```python
from build123d import *

# Parameters (mm, degrees)
ESQUISSE1_R             = 2.19
BOSS_EXTRU_2_DEPTH      = 3
ESQUISSE1_W             = 22.82
ESQUISSE1_H             = 8.5
BOSS_EXTRU_2_2_DEPTH    = 3
BOSS_EXTRU_4_DEPTH      = 3
CONG_1_R                = 3
ESQUISSE4_W             = 3
ESQUISSE4_H             = 9.614426754
BOSS_EXTRU_5_DEPTH      = 5
ENL_V_MAT_EXTRU_1_DEPTH = 5
ESQUISSE15_W            = 3
ESQUISSE15_H            = 34.885573246
BOSS_EXTRU_6_DEPTH      = 22.8
ESQUISSE17_R            = 1.25
ENL_V_MAT_EXTRU_2_DEPTH = 4
ESQUISSE19_R            = 2.5
ENL_V_MAT_EXTRU_5_DEPTH = 4


with BuildPart() as part:
    # Esquisse1 → Boss.-Extru.2 (new body)
    with BuildSketch(Plane.XY):
        Polygon((-22.134709342, 12.031312967), (-22.134709342, 3.531312967), (-2.314709342, 3.531312967), (-2.314709342, 2.416886213), (0.685290658, 2.416886213), (0.685290658, 12.031312967), align=None)
        with Locations((-17.224709342, 6.731312967)):
            Circle(ESQUISSE1_R, mode=Mode.SUBTRACT)
        with Locations((-7.224709342, 6.731312967)):
            Circle(ESQUISSE1_R, mode=Mode.SUBTRACT)
    extrude(amount=BOSS_EXTRU_2_DEPTH)



with BuildPart() as body_2:
    # Esquisse1 → Boss.-Extru.2 2 (new body)
    with BuildSketch(Plane.XY):
        with Locations((-10.724709342, -42.718687033)):
            Rectangle(ESQUISSE1_W, ESQUISSE1_H)
        with Locations((-17.224709342, -41.668687033)):
            Circle(ESQUISSE1_R, mode=Mode.SUBTRACT)
        with Locations((-7.224709342, -41.668687033)):
            Circle(ESQUISSE1_R, mode=Mode.SUBTRACT)
    extrude(amount=BOSS_EXTRU_2_2_DEPTH)

    # Esquisse3 → Boss.-Extru.4 (add)
    with BuildSketch(Plane(origin=(0.685290658, 0, 0), x_dir=(0, 0, -1), z_dir=(1, 0, 0))):
        with BuildLine():
            Line((0, 2.416886213), (0, 12.031312967))
            Line((0, 12.031312967), (-31.7, 12.031312967))
            Line((-31.7, 12.031312967), (-31.7, -46.968687033))
            Line((-31.7, -46.968687033), (0, -46.968687033))
            Line((0, -46.968687033), (0, -38.468687033))
            Line((0, -38.468687033), (-3, -38.468687033))
            ThreePointArc((-3, -38.468687033), (-4.5, -36.968687033), (-3, -35.468687033))
            Line((-3, -35.468687033), (5, -35.468687033))
            Line((5, -35.468687033), (5, -0.583113787))
            Line((5, -0.583113787), (-3, -0.583113787))
            ThreePointArc((-3, -0.583113787), (-4.5, 0.916886213), (-3, 2.416886213))
            Line((-3, 2.416886213), (0, 2.416886213))
        make_face()
    extrude(amount=BOSS_EXTRU_4_DEPTH)

    # Congé1
    cong_1_edges = [body_2.edges().sort_by_distance(p)[0] for p in [
        (2.185290658, -35.468687033, -5),
        (2.185290658, -0.583113787, -5),
    ]]
    fillet(cong_1_edges, radius=CONG_1_R)


with BuildPart() as part_1:
    add(part.part)

    add(body_2.part)  # Boss.-Extru.5 merges body 2
    # Esquisse4 → Boss.-Extru.5 (add)
    with BuildSketch(Plane(origin=(3.685290658, 0, 0), x_dir=(0, 0, -1), z_dir=(1, 0, 0))):
        with Locations((-1.5, 7.22409959)):
            Rectangle(ESQUISSE4_W, ESQUISSE4_H)
    extrude(amount=-BOSS_EXTRU_5_DEPTH)

    # Esquisse13 → Enlèv. mat.-Extru.1 (cut)
    with BuildSketch(Plane.ZY.offset(-0.685290658)):
        Polygon((28.7, -0.583113787), (31.7, -0.583113787), (31.7, 12.031312967), (24.585573245, 12.031312967), (24.585573245, 3.531312967), (28.7, 3.531312967), align=None)
        with BuildLine():
            ThreePointArc((28.7, -0.583113787), (25.790660941, 0.621973908), (24.585573245, 3.531312967))
            Line((24.585573245, 3.531312967), (28.7, 3.531312967))
            Line((28.7, 3.531312967), (28.7, -0.583113787))
        make_face()
        Polygon((31.7, -46.968687033), (31.7, -35.468687033), (28.7, -35.468687033), (28.7, -38.468687033), (25.7, -38.468687033), (25.7, -46.968687033), align=None)
        with BuildLine():
            ThreePointArc((25.7, -38.468687033), (26.578679656, -36.347366689), (28.7, -35.468687033))
            Line((28.7, -35.468687033), (28.7, -38.468687033))
            Line((28.7, -38.468687033), (25.7, -38.468687033))
        make_face()
    extrude(amount=-ENL_V_MAT_EXTRU_1_DEPTH, mode=Mode.SUBTRACT)

    # Esquisse15 → Boss.-Extru.6 (add)
    with BuildSketch(Plane.ZY.offset(-0.685290658)):
        with Locations((30.2, -18.02590041)):
            Rectangle(ESQUISSE15_W, ESQUISSE15_H)
    extrude(amount=BOSS_EXTRU_6_DEPTH)

    # Esquisse17 → Enlèv. mat.-Extru.2 (cut)
    with BuildSketch(Plane(origin=(3.685290658, 0, 0), x_dir=(0, 0, -1), z_dir=(1, 0, 0))):
        with Locations((-20.861566887, -16.89090041)):
            Circle(ESQUISSE17_R)
        with Locations((-20.861566887, -24.89090041)):
            Circle(ESQUISSE17_R)
        with Locations((-12.861566887, -24.89090041)):
            Circle(ESQUISSE17_R)
        with Locations((-4.861566887, -24.89090041)):
            Circle(ESQUISSE17_R)
        with Locations((-4.861566887, -16.89090041)):
            Circle(ESQUISSE17_R)
        with Locations((-4.861566887, -8.89090041)):
            Circle(ESQUISSE17_R)
        with Locations((-12.861566887, -8.89090041)):
            Circle(ESQUISSE17_R)
        with Locations((-20.861566887, -8.89090041)):
            Circle(ESQUISSE17_R)
        with Locations((-12.861566887, -0.89090041)):
            Circle(ESQUISSE17_R)
        with Locations((-12.861566887, -32.89090041)):
            Circle(ESQUISSE17_R)
        with Locations((-12.861566887, -16.89090041)):
            Circle(ESQUISSE17_R)
    extrude(amount=-ENL_V_MAT_EXTRU_2_DEPTH, mode=Mode.SUBTRACT)

    # Esquisse19 → Enlèv. mat.-Extru.5 (cut)
    with BuildSketch(Plane.XY.offset(31.7)):
        with Locations((-12.214709342, -6.873113787)):
            Circle(ESQUISSE19_R)
        with Locations((-12.214709342, -29.178687033)):
            Circle(ESQUISSE19_R)
    extrude(amount=-ENL_V_MAT_EXTRU_5_DEPTH, mode=Mode.SUBTRACT)


solid = part_1.part
```
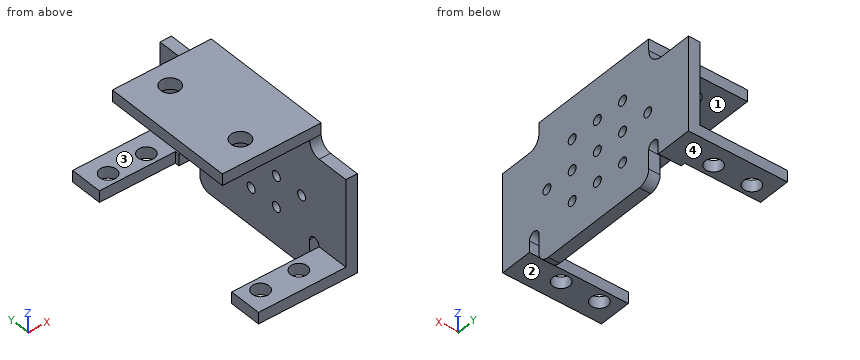
Geometry: final body of the model. Coordinates: model frame, mm. Face numbers are marked on the shaded views. A direction names the side the tool comes from. Coordinates: 2 decimals unless noted, no trailing zeros. Order: outer loops, then holes, each group sorted by start corner. A loop starts at its lowest first (then second) coordinate and runs counter-clockwise, first axis right, second up. Notation, with made-up numbers: (8.5, 85) -> (14.5, 85) arc R24 ccw to (14.5, 100) -> close; hole circle Ø6 at (58, 23). An arc over 180 degrees is marked (long way). Write item = value, one per line.
(1) Cut plane C-C on x = -20.5. Return loops of the section in (y, z), plus the area to 3 significant figures.
Solved:
outline = (-46.97, 0) -> (-38.47, 0) -> (-38.47, 3) -> (-46.97, 3) -> close; (-35.47, 28.7) -> (-0.58, 28.7) -> (-0.58, 31.7) -> (-35.47, 31.7) -> close; (3.53, 0) -> (12.03, 0) -> (12.03, 3) -> (3.53, 3) -> close
area = 156 mm²
(2) Cut plane D-D on y = -22. Return loops of the section in (x, z).
Solved:
outline = (-22.11, 28.7) -> (0.69, 28.7) -> (0.69, -5) -> (3.69, -5) -> (3.69, 31.7) -> (-22.11, 31.7) -> close
(3) Pin query (flat end, axial travel): pin 1 Ø3.5 at (x, y) = (-17.22, 6.73) entering from +Z; pin 2 Ø9.5 at (x, y) = (-13, -41) entering from -Z; pin 3 Ø10 at (x, y) = (-14, -11.5) entering from -Z; pin 4 Ø1.5 at (y, z) = (-24.5, 17.5) entering from -X. Return the tip coordinate at first contact, or that it passes through.
Solved:
pin_1 = through
pin_2 = 0
pin_3 = 28.7
pin_4 = 0.69
(4) Access query for the marked faces 1, 2, 3 and 4. Directions: +Z, -Z, +X, -X, +Y, -Y. A direction counts if a zero-diameter tool reaches every point of the face in a straight line with its end or side. Return the directions, or none.
Solved:
face_1 = -Z, -X, +Y, -Y
face_2 = -Z, +X, -X, -Y
face_3 = +Z, -X, +Y, -Y
face_4 = -Z, +X, -X, +Y
(5) Line query: line 1 (Y direction, x = -16, z = 1); line 2 (X direction, y = -10, z = -1); line 3 (Z direction, x = -19.25, y = -10.5). Output: solid intervals per line, ascending.
Solved:
line_1 = -46.97 to -43.48, -39.85 to -38.47, 3.53 to 4.92, 8.55 to 12.03
line_2 = 0.69 to 3.69
line_3 = 28.7 to 31.7
(6) Cut plane B-B on x = -6.5. Return loops of the section in (y, z).
Solved:
outline = (-46.97, 0) -> (-43.74, 0) -> (-43.74, 3) -> (-46.97, 3) -> close; (-39.6, 0) -> (-38.47, 0) -> (-38.47, 3) -> (-39.6, 3) -> close; (-35.47, 28.7) -> (-0.58, 28.7) -> (-0.58, 31.7) -> (-35.47, 31.7) -> close; (3.53, 0) -> (4.66, 0) -> (4.66, 3) -> (3.53, 3) -> close; (8.8, 0) -> (12.03, 0) -> (12.03, 3) -> (8.8, 3) -> close
(7) Cut plane A-A on z = 2. Return loops of the section in (x, y), plus the area to 3 significant figures.
Solved:
outline = (-22.13, -46.97) -> (3.69, -46.97) -> (3.69, -38.47) -> (-22.13, -38.47) -> close; (-22.13, 3.53) -> (-2.31, 3.53) -> (-2.31, 2.42) -> (3.69, 2.42) -> (3.69, 12.03) -> (-22.13, 12.03) -> close; (0.69, -35.47) -> (3.69, -35.47) -> (3.69, -0.58) -> (0.69, -0.58) -> close; hole circle Ø4.38 at (-17.22, -41.67); hole circle Ø4.38 at (-17.22, 6.73); hole circle Ø4.38 at (-7.22, -41.67); hole circle Ø4.38 at (-7.22, 6.73)
area = 490 mm²
